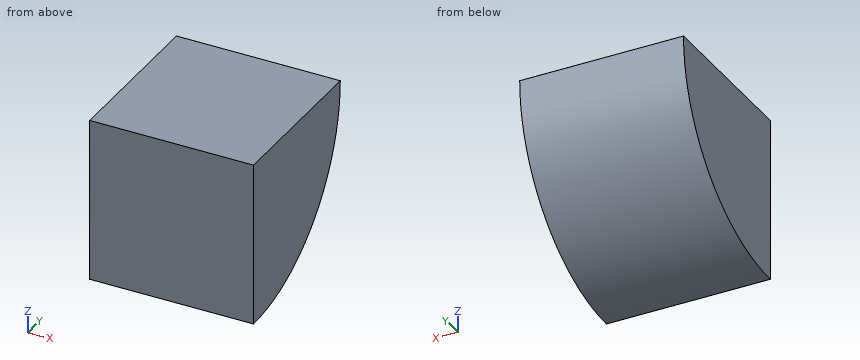
Autodesk Inventor part; units mm, degrees
ref_plane "YZ Plane" through (0, 0, 0) normal (1, 0, 0) x (0, 1, 0)
ref_plane "XZ Plane" through (0, 0, 0) normal (0, 1, 0) x (-1, 0, 0)
ref_plane "XY Plane" through (0, 0, 0) normal (0, 0, 1) x (1, 0, 0)
sketch "Skizze1" plane through (0, 0, 0) normal (0, 0, 1) x (1, 0, 0)
  line L0 (-9.6, 0) -> (1.6, 0)
  line L1 (0, -9.6) -> (0, 1.6)
  line L2 (0, 0) -> (-8, 0)
  line L3 (-8, 0) -> (-8, -8)
  line L4 (-8, -8) -> (0, -8)
  line L5 (0, -8) -> (0, 0)
  point P0 (0, -8)
  point P1 (-8, 0)
  point P2 (0, -8)
  dimension "d0" = 8
  dimension "d1" = 8
extrude "Extrusion1" add sketch "Skizze1" along normal blind 8
fillet "Rundung2" radius 8 1 edges at (-4, 0, 0)
properties part number "Eihalter_Halter" material "Acetalharz, Schwarz"
Design review of the part built by this model. Coordinates are the model's own, in mm. Coordinates: 2 decimals unless noted, no trailing zeros. Loops run counter-clockwise (first coordinate to the right, second up) from the corner with the lowest first, then second, coordinate; pieces in that order, holes last.
Item 1: Wall thickness on L1, parallel to Z at x = -4.5, y = -0.75; L2, parallel to Y at x = -5, z = 4.75; L3, parallel to Z at x = -5.5, y = -3: over which ranges is each line inside the solid? List them lowest first.
Completed:
L1: z = 4.62 to 8
L2: y = -8 to -0.69
L3: z = 1.75 to 8
Item 2: Add section B-B (z = 5.25). Write out the cut boundary in (x, y).
Completed:
outline: (-8, -8) - (0, -8) - (0, -0.49) - (-8, -0.49) - close
Item 3: Clearance check with flat-ended pins moving along their axes: pin 1 (1 mm diameter, centred on x = -5.5, y = -3, fed in from -Z); pin 2 (3 mm diameter, centred on y = -3, z = 1, fed in from +X). State where each tip first meets the part, or that it passes through.
Completed:
pin 1: stops at z = 1.39
pin 2: stops at x = 0
Item 4: Add section C-C (y = -2.75). Write out the cut boundary in (x, z), and give its area (3 significant figures).
Completed:
outline: (-8, 1.96) - (0, 1.96) - (0, 8) - (-8, 8) - close
area: 48.3 mm2
